For this review, take the finished solid that the model builds, in its own axes (mm). Face numbers are marked on the shaded views. A direction names the side the tool comes from. Round coordinates to 2 decimals unless told otherwise and drop trailing zeros. Order: outer loops, then holes, each group sorted by start corner. A loop starts at its lowest first (then second) coordinate and runs counter-clockwise, first axis right, second up. Notation, with made-up numbers: (-8, -37) - (5, -37) arc R23 cw to (5, -25) - close; hole circle Ø1 at (70, 61). An arc over 180 degrees is marked (long way). One line per question, with ' | ' between items.
```python
from build123d import *

# Parameters (mm, degrees)
F0_W     = 8
F0_H     = 153
F1_DEPTH = 7
F3_DEPTH = 160
F4_W     = 8
F4_H     = 179
F5_DEPTH = 1
F6_R     = 0.99999


# Not quite as in the source:
# - a fillet or chamfer is up to 0.001 mm smaller than in the source, because OpenCascade refuses the exact size


with BuildPart() as f1:
    # F0 (on Top) → F1 (new body)
    with BuildSketch(Plane.XY):
        Rectangle(F0_W, F0_H)
    extrude(amount=F1_DEPTH)

    # F2 (on face) → F3 (cut)
    with BuildSketch(Plane.XZ.offset(76.5)):
        with BuildLine():
            Line((4, 7), (-2, 7))
            ThreePointArc((-2, 7), (-0.1605232856, 3.1073720572), (4, 2))
            Line((4, 2), (4, 7))
        make_face()
    extrude(amount=-F3_DEPTH, mode=Mode.SUBTRACT)

    # F4 (on face) → F5 (join)
    with BuildSketch(Plane(origin=(0, 0, 0), x_dir=(1, 0, 0), z_dir=(0, 0, -1))):
        Rectangle(F4_W, F4_H)
    extrude(amount=F5_DEPTH)

    # F6 (radius 1 in the source; OpenCascade refuses exactly that, so slightly less here)
    f6_edges = [f1.edges().sort_by_distance(p)[0] for p in [
        (0, -89.5, 0),
        (0, 89.5, 0),
    ]]
    fillet(f6_edges, radius=F6_R)


solid = f1.part
```
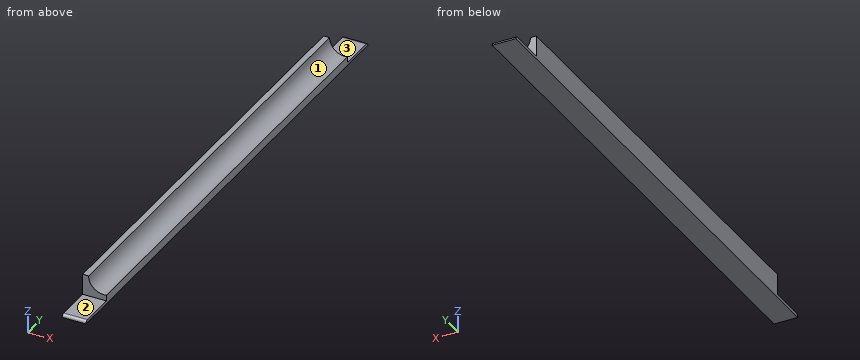
(1) Insertion check: pin 1 (1 mm diameter, centred on x = 0.5, z = 1.5, fed in from +Y); pin 2 (1 mm diameter, centred on x = -3, z = 2, fed in from -Y); pin 3 (2 mm diameter, centred on x = 0.5, y = -32.5, fed in from +Z). Each pin has a flat end and moves straight along its axis. Give the tip position at first contact, or say it passes through.
Output values:
pin 1: y = 76.5 | pin 2: y = -76.5 | pin 3: z = 3.42
(2) For the marked faces 1, 2 and 3, list the 3-axis set-ups (+Z, -Z, +X, -X, +Y, -Y) from which the entire face can be reached by the end or side of a thin tool; tool diameter is ignored.
Output values:
face 1: +Z, +Y, -Y | face 2: +Z, +X, -X, -Y | face 3: +Z, +X, -X, +Y
(3) We need section B-B on y = 38.5. State the section outline as (x, z) points.
Output values:
outline: (-4, -1) - (4, -1) - (4, 2) arc R5.11 cw to (-2, 7) - (-4, 7) - close
(4) For probe 1 along Y at (x, z) = (-3.5, 5); probe 2 along Z at (x, y) = (2.25, 78.5); probe 3 along Z at (x, y) = (3.25, -39), list the stretches that pass through material, from the lowest coordinate up. Write a range as [from, to].
Output values:
probe 1: [-76.5, 76.5] | probe 2: [-1, 0] | probe 3: [-1, 1.92]
(5) We need section C-C on z = 4.75. State the section outline as (x, y) points, plus the area to 3 significant figures.
Output values:
outline: (-4, -76.5) - (-1.46, -76.5) - (-1.46, 76.5) - (-4, 76.5) - close | area: 388 mm^2
